```python
from build123d import *

# Parameters (mm, degrees)
SKETCH1_W                 = 13
SKETCH1_H                 = 16
BOSS_EXTRUDE1_DEPTH       = 4
SKETCH2_R                 = 1.65
CUT_EXTRUDE1_DEPTH        = 10
SKETCH3_W                 = 4
SKETCH3_H                 = 13
BOSS_EXTRUDE2_DEPTH       = 4
SKETCH4_W                 = 13
SKETCH4_H                 = 4
BOSS_EXTRUDE3_DEPTH       = 60
SKETCH6_W                 = 4
SKETCH6_H                 = 21
SKETCH6_H_2               = 13
BOSS_EXTRUDE4_DEPTH       = 28
SKETCH12_W                = 4
SKETCH12_H                = 28
BOSS_EXTRUDE8_DEPTH       = 1.65
SKETCH13_W                = 4
SKETCH13_H                = 28
BOSS_EXTRUDE9_DEPTH       = 1.65
SKETCH14_W                = 4
SKETCH14_H                = 35.878399396
CUT_EXTRUDE5_DEPTH        = 24
SKETCH15_R                = 1.65
CUT_EXTRUDE6_DEPTH        = 24
SKETCH16_W                = 4
SKETCH16_H                = 11.121600604
SKETCH16_H_2              = 11.3
BOSS_EXTRUDE10_DEPTH      = 29.15
SKETCH17_R                = 1.65
CUT_EXTRUDE8_DEPTH        = 29.15
SKETCH18_W                = 22.65
SKETCH18_H                = 4
SKETCH18_W_2              = 13
BOSS_EXTRUDE11_DEPTH      = 4
SKETCH19_W                = 4
SKETCH19_H                = 20
BOSS_EXTRUDE12_DEPTH      = 40
SKETCH20_R                = 1.65
CUT_EXTRUDE9_DEPTH        = 40
SKETCH21_W                = 4
SKETCH21_H                = 30.5
BOSS_EXTRUDE13_DEPTH      = 38.5
SKETCH23_W                = 4
SKETCH23_H                = 4
BOSS_EXTRUDE14_DEPTH      = 38.5
SKETCH24_W                = 4
SKETCH24_H                = 38.5
BOSS_EXTRUDE15_DEPTH      = 3
SKETCH27_W                = 4
SKETCH27_H                = 58.3
CUT_EXTRUDE10_DEPTH       = 100
SKETCH29_W                = 38.5
SKETCH29_H                = 7
BOSS_EXTRUDE16_DEPTH      = 40
BOSS_EXTRUDE16_DEPTH_BACK = 28
SKETCH30_R                = 1.65
CUT_EXTRUDE11_DEPTH       = 40
SKETCH31_W                = 4
SKETCH31_H                = 22.5
CUT_EXTRUDE12_DEPTH       = 38.5
SKETCH32_W                = 38.5
SKETCH32_H                = 2.5
CUT_EXTRUDE13_DEPTH       = 40
SKETCH33_W                = 4
SKETCH33_H                = 8
BOSS_EXTRUDE17_DEPTH      = 8
SKETCH34_R                = 1.65
CUT_EXTRUDE14_DEPTH       = 8
SKETCH35_W                = 4
SKETCH35_H                = 43.5
BOSS_EXTRUDE18_DEPTH      = 13
CUT_EXTRUDE15_START       = -20
SKETCH36_W                = 10
SKETCH36_H                = 80
CUT_EXTRUDE15_DEPTH       = 20
SKETCH37_W                = 5
SKETCH37_H                = 7
BOSS_EXTRUDE19_DEPTH      = 4
SKETCH41_W                = 13
SKETCH41_H                = 20
BOSS_EXTRUDE20_DEPTH      = 4
SKETCH42_R                = 1.65
CUT_EXTRUDE18_DEPTH       = 4
SKETCH43_W                = 4
SKETCH43_H                = 38.5
CUT_EXTRUDE19_DEPTH       = 10
SKETCH44_W                = 8
SKETCH44_H                = 9
BOSS_EXTRUDE21_DEPTH      = 4
SKETCH45_R                = 1.65
CUT_EXTRUDE20_DEPTH       = 4
CUT_EXTRUDE21_DEPTH       = 3
SKETCH49_R                = 1.65
CUT_EXTRUDE22_DEPTH       = 5
SKETCH54_W                = 1
SKETCH54_H                = 38.5
CUT_EXTRUDE24_DEPTH       = 50


with BuildPart() as part:
    # Sketch1 → Boss-Extrude1 (new body)
    with BuildSketch(Plane(origin=(0, 0, 0), x_dir=(0, 0, -1), z_dir=(1, 0, 0))):
        with Locations((6.5, -8)):
            Rectangle(SKETCH1_W, SKETCH1_H)
    extrude(amount=BOSS_EXTRUDE1_DEPTH)

    # Sketch2 → Cut-Extrude1 (cut)
    with BuildSketch(Plane(origin=(4, 0, 0), x_dir=(0, 0, -1), z_dir=(1, 0, 0))):
        with Locations((6.5, -4)):
            Circle(SKETCH2_R)
        with Locations((6.5, -12)):
            Circle(SKETCH2_R)
    extrude(amount=-CUT_EXTRUDE1_DEPTH, mode=Mode.SUBTRACT)

    # Sketch3 → Boss-Extrude2 (add)
    with BuildSketch(Plane.XZ.offset(16)):
        with Locations((2, -6.5)):
            Rectangle(SKETCH3_W, SKETCH3_H)
    extrude(amount=BOSS_EXTRUDE2_DEPTH)

    # Sketch4 → Boss-Extrude3 (add)
    with BuildSketch(Plane(origin=(4, 0, 0), x_dir=(0, 0, -1), z_dir=(1, 0, 0))):
        with Locations((6.5, -18)):
            Rectangle(SKETCH4_W, SKETCH4_H)
    extrude(amount=BOSS_EXTRUDE3_DEPTH)

    # Sketch6 → Boss-Extrude4 (add)
    with BuildSketch(Plane(origin=(0, -16, 0), x_dir=(1, 0, 0), z_dir=(0, 1, 0))):
        with Locations((62, -10.5)):
            Rectangle(SKETCH6_W, SKETCH6_H)
        with Locations((62, 23.5)):
            Rectangle(SKETCH6_W, SKETCH6_H)
        with Locations((62, 6.5)):
            Rectangle(SKETCH6_W, SKETCH6_H_2)
    extrude(amount=BOSS_EXTRUDE4_DEPTH)

    # Sketch12 → Boss-Extrude8 (add)
    with BuildSketch(Plane(origin=(0, 0, -34), x_dir=(-1, 0, 0), z_dir=(0, 0, -1))):
        with Locations((-62, -2)):
            Rectangle(SKETCH12_W, SKETCH12_H)
    extrude(amount=BOSS_EXTRUDE8_DEPTH)

    # Sketch13 → Boss-Extrude9 (add)
    with BuildSketch(Plane.XY.offset(21)):
        with Locations((62, -2)):
            Rectangle(SKETCH13_W, SKETCH13_H)
    extrude(amount=BOSS_EXTRUDE9_DEPTH)

    # Sketch14 → Cut-Extrude5 (cut)
    with BuildSketch(Plane(origin=(0, 12, 0), x_dir=(1, 0, 0), z_dir=(0, 1, 0))):
        with Locations((62, 6.410800302)):
            Rectangle(SKETCH14_W, SKETCH14_H)
    extrude(amount=-CUT_EXTRUDE5_DEPTH, mode=Mode.SUBTRACT)

    # Sketch15 → Cut-Extrude6 (cut)
    with BuildSketch(Plane(origin=(64, 0, 0), x_dir=(0, 0, -1), z_dir=(1, 0, 0))):
        with Locations((-17, -11.5)):
            Circle(SKETCH15_R)
        with Locations((30, -11.5)):
            Circle(SKETCH15_R)
    extrude(amount=-CUT_EXTRUDE6_DEPTH, mode=Mode.SUBTRACT)

    # Sketch16 → Boss-Extrude10 (add)
    with BuildSketch(Plane(origin=(0, 12, 0), x_dir=(1, 0, 0), z_dir=(0, 1, 0))):
        with Locations((62, -17.089199698)):
            Rectangle(SKETCH16_W, SKETCH16_H)
        with Locations((62, 30)):
            Rectangle(SKETCH16_W, SKETCH16_H_2)
    extrude(amount=BOSS_EXTRUDE10_DEPTH)

    # Sketch17 → Cut-Extrude8 (cut)
    with BuildSketch(Plane(origin=(64, 0, 0), x_dir=(0, 0, -1), z_dir=(1, 0, 0))):
        with Locations((-17, 35.5)):
            Circle(SKETCH17_R)
        with Locations((30, 35.5)):
            Circle(SKETCH17_R)
    extrude(amount=-CUT_EXTRUDE8_DEPTH, mode=Mode.SUBTRACT)

    # Sketch18 → Boss-Extrude11 (add)
    with BuildSketch(Plane(origin=(64, 0, 0), x_dir=(0, 0, -1), z_dir=(1, 0, 0))):
        with Locations((-11.325, -18)):
            Rectangle(SKETCH18_W, SKETCH18_H)
        with Locations((24.325, -18)):
            Rectangle(SKETCH18_W, SKETCH18_H)
        with Locations((6.5, -18)):
            Rectangle(SKETCH18_W_2, SKETCH18_H)
    extrude(amount=-BOSS_EXTRUDE11_DEPTH)

    # Sketch19 → Boss-Extrude12 (add)
    with BuildSketch(Plane(origin=(0, 0, -13), x_dir=(-1, 0, 0), z_dir=(0, 0, -1))):
        with Locations((-2, -10)):
            Rectangle(SKETCH19_W, SKETCH19_H)
    extrude(amount=BOSS_EXTRUDE12_DEPTH)

    # Sketch20 → Cut-Extrude9 (cut)
    with BuildSketch(Plane.ZY):
        with Locations((-46.5, -4)):
            Circle(SKETCH20_R)
        with Locations((-46.5, -12)):
            Circle(SKETCH20_R)
    extrude(amount=-CUT_EXTRUDE9_DEPTH, mode=Mode.SUBTRACT)

    # Sketch21 → Boss-Extrude13 (add)
    with BuildSketch(Plane(origin=(0, -16, 0), x_dir=(1, 0, 0), z_dir=(0, 1, 0))):
        with Locations((26, 6.5)):
            Rectangle(SKETCH21_W, SKETCH21_H)
    extrude(amount=BOSS_EXTRUDE13_DEPTH)

    # Sketch23 → Boss-Extrude14 (add)
    with BuildSketch(Plane(origin=(0, 22.5, 0), x_dir=(1, 0, 0), z_dir=(0, 1, 0))):
        with Locations((26, 23.75)):
            Rectangle(SKETCH23_W, SKETCH23_H)
        with Locations((26, -10.75)):
            Rectangle(SKETCH23_W, SKETCH23_H)
    extrude(amount=-BOSS_EXTRUDE14_DEPTH)

    # Sketch24 → Boss-Extrude15 (add)
    with BuildSketch(Plane(origin=(0, 22.5, 0), x_dir=(1, 0, 0), z_dir=(0, 1, 0))):
        with Locations((26, 6.5)):
            Rectangle(SKETCH24_W, SKETCH24_H)
    extrude(amount=BOSS_EXTRUDE15_DEPTH)

    # Sketch27 → Cut-Extrude10 (cut)
    with BuildSketch(Plane.XZ.offset(20)):
        with Locations((62, -6.5)):
            Rectangle(SKETCH27_W, SKETCH27_H)
    extrude(amount=-CUT_EXTRUDE10_DEPTH, mode=Mode.SUBTRACT)

    # Sketch29 → Boss-Extrude16 (add, two sides)
    with BuildSketch(Plane(origin=(28, 0, 0), x_dir=(0, 0, -1), z_dir=(1, 0, 0))) as boss_extrude16_sk:
        with Locations((6.5, -16.5)):
            Rectangle(SKETCH29_W, SKETCH29_H)
    extrude(amount=BOSS_EXTRUDE16_DEPTH)
    extrude(boss_extrude16_sk.sketch, amount=-BOSS_EXTRUDE16_DEPTH_BACK)

    # Sketch30 → Cut-Extrude11 (cut)
    with BuildSketch(Plane.ZY.offset(-24)):
        with Locations((8.75, 21.5)):
            Circle(SKETCH30_R)
        with Locations((8.75, -9)):
            Circle(SKETCH30_R)
        with Locations((-21.75, 21.5)):
            Circle(SKETCH30_R)
        with Locations((-21.75, -9)):
            Circle(SKETCH30_R)
    extrude(amount=-CUT_EXTRUDE11_DEPTH, mode=Mode.SUBTRACT)

    # Sketch31 → Cut-Extrude12 (cut)
    with BuildSketch(Plane(origin=(0, 25.5, 0), x_dir=(1, 0, 0), z_dir=(0, 1, 0))):
        with Locations((26, 6.5)):
            Rectangle(SKETCH31_W, SKETCH31_H)
    extrude(amount=-CUT_EXTRUDE12_DEPTH, mode=Mode.SUBTRACT)

    # Sketch32 → Cut-Extrude13 (cut)
    with BuildSketch(Plane(origin=(68, 0, 0), x_dir=(0, 0, -1), z_dir=(1, 0, 0))):
        with Locations((6.5, -14.25)):
            Rectangle(SKETCH32_W, SKETCH32_H)
    extrude(amount=-CUT_EXTRUDE13_DEPTH, mode=Mode.SUBTRACT)

    # Sketch33 → Boss-Extrude17 (add)
    with BuildSketch(Plane(origin=(0, 25.5, 0), x_dir=(1, 0, 0), z_dir=(0, 1, 0))):
        with Locations((26, -8.75)):
            Rectangle(SKETCH33_W, SKETCH33_H)
        with Locations((26, 21.75)):
            Rectangle(SKETCH33_W, SKETCH33_H)
    extrude(amount=-BOSS_EXTRUDE17_DEPTH)

    # Sketch34 → Cut-Extrude14 (cut)
    with BuildSketch(Plane(origin=(28, 0, 0), x_dir=(0, 0, -1), z_dir=(1, 0, 0))):
        with Locations((-8.75, 21.5)):
            Circle(SKETCH34_R)
        with Locations((21.75, 21.5)):
            Circle(SKETCH34_R)
    extrude(amount=-CUT_EXTRUDE14_DEPTH, mode=Mode.SUBTRACT)

    # Sketch35 → Boss-Extrude18 (add)
    with BuildSketch(Plane(origin=(0, -13, 0), x_dir=(1, 0, 0), z_dir=(0, 1, 0))):
        with Locations((12, 9)):
            Rectangle(SKETCH35_W, SKETCH35_H)
    extrude(amount=BOSS_EXTRUDE18_DEPTH)

    # Sketch36 → Cut-Extrude15 (cut)
    with BuildSketch(Plane.XZ.offset(20).offset(CUT_EXTRUDE15_START)):
        with Locations((5, -27.25)):
            Rectangle(SKETCH36_W, SKETCH36_H)
    extrude(amount=CUT_EXTRUDE15_DEPTH, mode=Mode.SUBTRACT)

    # Sketch37 → Boss-Extrude19 (add)
    with BuildSketch(Plane.ZY.offset(-10)):
        with Locations((-28.25, -16.5)):
            Rectangle(SKETCH37_W, SKETCH37_H)
    extrude(amount=-BOSS_EXTRUDE19_DEPTH)

    # Sketch41 → Boss-Extrude20 (add)
    with BuildSketch(Plane(origin=(14, 0, 0), x_dir=(0, 0, -1), z_dir=(1, 0, 0))):
        with Locations((32.25, -10)):
            Rectangle(SKETCH41_W, SKETCH41_H)
    extrude(amount=-BOSS_EXTRUDE20_DEPTH)

    # Sketch42 → Cut-Extrude18 (cut)
    with BuildSketch(Plane.ZY.offset(-10)):
        with Locations((-32.25, -4)):
            Circle(SKETCH42_R)
        with Locations((-32.25, -12)):
            Circle(SKETCH42_R)
    extrude(amount=-CUT_EXTRUDE18_DEPTH, mode=Mode.SUBTRACT)

    # Sketch43 → Cut-Extrude19 (cut)
    with BuildSketch(Plane(origin=(0, 0, 0), x_dir=(1, 0, 0), z_dir=(0, 1, 0))):
        with Locations((12, 6.5)):
            Rectangle(SKETCH43_W, SKETCH43_H)
    extrude(amount=-CUT_EXTRUDE19_DEPTH, mode=Mode.SUBTRACT)

    # Sketch44 → Boss-Extrude21 (add)
    with BuildSketch(Plane(origin=(28, 0, 0), x_dir=(0, 0, -1), z_dir=(1, 0, 0))):
        with Locations((-8.75, -11)):
            Rectangle(SKETCH44_W, SKETCH44_H)
        with Locations((21.75, -11)):
            Rectangle(SKETCH44_W, SKETCH44_H)
    extrude(amount=-BOSS_EXTRUDE21_DEPTH)

    # Sketch45 → Cut-Extrude20 (cut)
    with BuildSketch(Plane.ZY.offset(-24)):
        with Locations((-21.75, -7)):
            Circle(SKETCH45_R)
        with Locations((8.75, -7)):
            Circle(SKETCH45_R)
    extrude(amount=-CUT_EXTRUDE20_DEPTH, mode=Mode.SUBTRACT)

    # Sketch46 → Cut-Extrude21 (cut)
    with BuildSketch(Plane(origin=(0, -15.5, 0), x_dir=(1, 0, 0), z_dir=(0, 1, 0))):
        Polygon((64, 18.285898385), (67, 20.017949192), (67, 23.482050808), (64, 25.214101615), (61, 23.482050808), (61, 20.017949192), align=None)
        Polygon((64, -12.214101615), (67, -10.482050808), (67, -7.017949192), (64, -5.285898385), (61, -7.017949192), (61, -10.482050808), align=None)
    extrude(amount=-CUT_EXTRUDE21_DEPTH, mode=Mode.SUBTRACT)

    # Sketch49 → Cut-Extrude22 (cut)
    with BuildSketch(Plane(origin=(0, -15.5, 0), x_dir=(1, 0, 0), z_dir=(0, 1, 0))):
        with Locations((64, 21.75)):
            Circle(SKETCH49_R)
        with Locations((64, -8.75)):
            Circle(SKETCH49_R)
    extrude(amount=-CUT_EXTRUDE22_DEPTH, mode=Mode.SUBTRACT)

    # Sketch54 → Cut-Extrude24 (cut)
    with BuildSketch(Plane(origin=(0, -10, 0), x_dir=(1, 0, 0), z_dir=(0, 1, 0))):
        with Locations((10.5, 6.5)):
            Rectangle(SKETCH54_W, SKETCH54_H)
    extrude(amount=-CUT_EXTRUDE24_DEPTH, mode=Mode.SUBTRACT)


solid = part.part
```
Geometry check sheet. Reference: the model listing, model coordinates, mm. A direction names the side the tool comes from. Round coordinates to 2 decimals unless told otherwise and drop trailing zeros. Loops run counter-clockwise (first coordinate to the right, second up) from the corner with the lowest first, then second, coordinate; pieces in that order, holes last. Notation, with made-up numbers: M -31,47.5 L 13,47.5 A28 cw 13,78.5 Z; hole C 28.25,81.25 d8. An arc over 180 degrees is marked long. Return JSON: item names as keys, results as strings. Group by question number.
(1) Go/stop test with flat-tipped pins: pin 1 (1 mm diameter, centred on y = 6, z = -20.5, fed in from -X); pin 2 (4 mm diameter, centred on y = -12, z = -32.25, fed in from +X); pin 3 (3 mm diameter, centred on x = 12.5, y = -7, fed in from +Z); pin 4 (4 mm diameter, centred on x = 64, z = 8.75, fed in from -Y). Record where each tip stops, or that it passes through.
(2) Scan lines: line 1 along Y through (x, z) = (26.9, 8.75); line 2 along Z through (x, y) = (25, 21); line 3 along Z through (x, y) = (24.5, -10). Record each from-to range of solid material in increasing order. Write a range as [from, to].
(3) Mould release check, pull along X, two halves, no side actions. Record for faces 5 (the face through (10, -10, -32)), 6 (the face through (26.028, 22.615, -20.534)), 7 (the face through (62.35, -19.24, 8.68)): pulls with the +X half, pulls with the -X half, needs draft (parallel to the pull), parting line crosses it, or undercut.
(4) Section check C-C, the plane y = -7. Enter the section's corners in (x, z), and give its area (3 significant figures).
(5) Section check B-B, the plane z = -32.25. Enter the section's corners in (x, y).
(6) Set-up check for faces 1 (the face through (14, -11, -25)), 2 (the face through (35, -16, -25.75)), 3 (the face through (12, 0, -32)), 4 (the face through (65.521, -16.979, -24.336)): record each of +Z, -Z, +X, -X, +Y, -Y from which the full face is reachable in a straight line by a thin tool's end or side.
(7) Section check A-A, the plane y = 2.5. Enter the section's corners in (x, z).
(8) Section check D-D, the plane z = 8.75. Enter the section's corners in (x, y), and give its area (3 significant figures).
Data:
{
 "1": {"pin 1": "x = 24", "pin 2": "x = 14", "pin 3": "z = -25.75", "pin 4": "y = -20"},
 "2": {"line 1": "[-20, -8.65], [-5.35, 19.85], [23.15, 25.5]", "line 2": "[-25.75, -23.32], [-20.18, -17.75], [4.75, 7.18], [10.32, 12.75]", "line 3": "[-25.75, -17.75], [4.75, 12.75]"},
 "3": {"face 5": "pulls with the -X half", "face 6": "needs draft", "face 7": "undercut"},
 "4": {"outline": "M 10,-38.75 L 14,-38.75 L 14,-25.75 L 10,-25.75 Z; M 24,-25.75 L 28,-25.75 L 28,-23.4 L 24,-23.4 Z; M 24,-20.1 L 28,-20.1 L 28,-17.75 L 24,-17.75 Z; M 24,4.75 L 28,4.75 L 28,7.1 L 24,7.1 Z; M 24,10.4 L 28,10.4 L 28,12.75 L 24,12.75 Z", "area": "89.6 mm²"},
 "5": {"outline": "M 10,-20 L 14,-20 L 14,-13.65 L 10,-13.65 Z; M 10,-10.35 L 14,-10.35 L 14,-5.65 L 10,-5.65 Z; M 10,-2.35 L 14,-2.35 L 14,0 L 10,0 Z"},
 "6": {"face 1": "-Z, +Y", "face 2": "-Z, +X, +Y, -Y", "face 3": "+Z, -Z, +X, -X, +Y", "face 4": "+Y"},
 "7": {"outline": "M 24,-25.75 L 28,-25.75 L 28,-17.75 L 24,-17.75 Z; M 24,4.75 L 28,4.75 L 28,12.75 L 24,12.75 Z"},
 "8": {"outline": "M 11,-20 L 62.35,-20 L 62.35,-18.5 L 61,-18.5 L 61,-15.5 L 28,-15.5 L 28,-8.65 L 24,-8.65 L 24,-13 L 14,-13 L 14,-10 L 11,-10 Z; M 24,-5.35 L 28,-5.35 L 28,19.85 L 24,19.85 Z; M 24,23.15 L 28,23.15 L 28,25.5 L 24,25.5 Z; M 65.65,-20 L 68,-20 L 68,-15.5 L 67,-15.5 L 67,-18.5 L 65.65,-18.5 Z", "area": "413 mm²"}
}
